Geometry: final body of the model. Coordinates: model frame, mm. Give positions to 0.01 mm unless a question says otherwise; leave off trailing zeros. Write each loop counter-clockwise with the first axis right and the second up, starting at its lowest first coordinate (ties: lowest second). Pieces come first, ordered by that corner, then holes. Notation, with made-up numbers: (-32, -13.75) -> (2, -13.75) arc R29 ccw to (2, 13.25) -> close; hole circle Ø1 at (71.25, 16). An arc over 180 degrees is marked (long way). Answer as a JSON object with one key per item and string values.
from build123d import *

# Parameters (mm, degrees)
SKETCH1_W           = 15.5
SKETCH1_H           = 27.94
BOSS_EXTRUDE1_DEPTH = 1.6
SKETCH2_R           = 0.5
SKETCH2_R_2         = 1.778
CUT_EXTRUDE1_DEPTH  = 2
SKETCH3_R           = 0.2
CUT_EXTRUDE2_DEPTH  = 10


with BuildPart() as part:
    # Sketch1 → Boss-Extrude1 (new body)
    with BuildSketch(Plane.XY):
        Rectangle(SKETCH1_W, SKETCH1_H)
    extrude(amount=BOSS_EXTRUDE1_DEPTH)

    # Sketch2 → Cut-Extrude1 (cut)
    with BuildSketch(Plane.XY.offset(1.6)):
        with Locations((-6.48, -12.7)):
            Circle(SKETCH2_R)
        with Locations((-6.48, -10.16)):
            Circle(SKETCH2_R)
        with Locations((-6.48, -7.62)):
            Circle(SKETCH2_R)
        with Locations((-6.48, -5.08)):
            Circle(SKETCH2_R)
        with Locations((-6.48, -2.54)):
            Circle(SKETCH2_R)
        with Locations((-6.48, 0)):
            Circle(SKETCH2_R)
        with Locations((-6.48, 2.54)):
            Circle(SKETCH2_R)
        with Locations((-6.48, 5.08)):
            Circle(SKETCH2_R)
        with Locations((-6.48, 7.62)):
            Circle(SKETCH2_R)
        with Locations((-6.48, 10.16)):
            Circle(SKETCH2_R)
        with Locations((-6.48, 12.7)):
            Circle(SKETCH2_R)
        with Locations((5.26414257, 11.423545933)):
            Circle(SKETCH2_R_2)
        with Locations((5.26414257, -11.464062499)):
            Circle(SKETCH2_R_2)
    extrude(amount=-CUT_EXTRUDE1_DEPTH, mode=Mode.SUBTRACT)

    # Sketch3 → Cut-Extrude2 (cut)
    with BuildSketch(Plane.XY.offset(1.6)):
        with Locations((-1.830670849, 1.202487627)):
            Circle(SKETCH3_R)
        with Locations((-0.302406534, 3.125566843)):
            Circle(SKETCH3_R)
        with Locations((1.486755487, 3.791476374)):
            Circle(SKETCH3_R)
        with Locations((3.836977644, 4.423555572)):
            Circle(SKETCH3_R)
        with Locations((3.975659184, -2.601471813)):
            Circle(SKETCH3_R)
        with Locations((2.659050244, -4.790940134)):
            Circle(SKETCH3_R)
        with Locations((-1.177453811, -6.944947611)):
            Circle(SKETCH3_R)
        with Locations((-1.205838194, -3.50049205)):
            Circle(SKETCH3_R)
    extrude(amount=-CUT_EXTRUDE2_DEPTH, mode=Mode.SUBTRACT)


solid = part.part
Q1. Material intervals for L1, parallel to X at y = 12.75, z = 0.65; L2, parallel to X at y = -10.25, z = 0.55; L3, parallel to Y at x = 2.75, z = 0.5, sorted ascending. Write a range as from..to.
Values:
{"L1": "-7.75..-6.98, -5.98..4.08, 6.45..7.75", "L2": "-7.75..-6.97, -5.99..3.97, 6.56..7.75", "L3": "-13.97..-4.97, -4.61..13.97"}
Q2. Cut plane A-A (y = 0). Return the cut outline in (x, z).
Values:
{"outline": "(-7.75, 0) -> (-6.98, 0) -> (-6.98, 1.6) -> (-7.75, 1.6) -> close; (-5.98, 0) -> (7.75, 0) -> (7.75, 1.6) -> (-5.98, 1.6) -> close"}
Q3. Mould query, pull axis X, two halves, no side actions, for faces 1 (the flat face through (7.75, 0, 1)), 2 (the flat face through (0, 13.97, 1)), 3 (the flat face through (-7.75, 0, 1)), 4 (the cylindrical face through (-6.88, 2.24, 0.81)). Classes: pulls with the +X half, pulls with the -X half, needs draft (parallel to the pull), parting line crosses it, or undercut.
Values:
{"face 1": "pulls with the +X half", "face 2": "needs draft", "face 3": "pulls with the -X half", "face 4": "undercut"}
Q4. Cut plane B-B (x = 6.5). Return the cut outline in (y, z).
Values:
{"outline": "(-13.97, 0) -> (-12.74, 0) -> (-12.74, 1.6) -> (-13.97, 1.6) -> close; (-10.19, 0) -> (10.15, 0) -> (10.15, 1.6) -> (-10.19, 1.6) -> close; (12.7, 0) -> (13.97, 0) -> (13.97, 1.6) -> (12.7, 1.6) -> close"}
Q5. Cut plane D-D (y = -10.16). Return the cut outline in (x, z), and give its area (3 significant figures).
Values:
{"outline": "(-7.75, 0) -> (-6.98, 0) -> (-6.98, 1.6) -> (-7.75, 1.6) -> close; (-5.98, 0) -> (4.06, 0) -> (4.06, 1.6) -> (-5.98, 1.6) -> close; (6.47, 0) -> (7.75, 0) -> (7.75, 1.6) -> (6.47, 1.6) -> close", "area": "19.3 mm²"}
Q6. Cut plane C-C (z = 1.35). State how many separate pieces and enclosed holes the cut face has, and give its area (3 significant figures).
Values:
{"separate pieces": "1", "enclosed holes": "21", "area": "404 mm²"}
